```python
from build123d import *

# Parameters (mm, degrees)
CROQUIS1_W              = 208
CROQUIS1_H              = 365
SALIENTE_EXTRUIR1_DEPTH = 2.5
CROQUIS2_W              = 34
CROQUIS2_H              = 30
SALIENTE_EXTRUIR2_DEPTH = 1
CROQUIS3_W              = 208
CROQUIS3_H              = 135
CORTAR_EXTRUIR1_DEPTH   = 4.5
SKETCH1_R               = 2
CUT_EXTRUDE1_DEPTH      = 2.5


with BuildPart() as part:
    # Croquis1 → Saliente-Extruir1 (new body)
    with BuildSketch(Plane(origin=(0, 0, 0), x_dir=(1, 0, 0), z_dir=(0, 1, 0))):
        Rectangle(CROQUIS1_W, CROQUIS1_H)
    extrude(amount=SALIENTE_EXTRUIR1_DEPTH)

    # Croquis2 → Saliente-Extruir2 (add)
    with BuildSketch(Plane(origin=(0, 0, 0), x_dir=(-1, 0, 0), z_dir=(0, -1, 0))):
        with Locations((87, -31.5)):
            Rectangle(CROQUIS2_W, CROQUIS2_H)
        with Locations((-87, -31.5)):
            Rectangle(CROQUIS2_W, CROQUIS2_H)
        with Locations((-87, 22.5)):
            Rectangle(CROQUIS2_W, CROQUIS2_H)
        with Locations((87, 22.5)):
            Rectangle(CROQUIS2_W, CROQUIS2_H)
    extrude(amount=SALIENTE_EXTRUIR2_DEPTH)

    # Croquis3 → Cortar-Extruir1 (cut, through all)
    with BuildSketch(Plane(origin=(0, 2.5, 0), x_dir=(1, 0, 0), z_dir=(0, 1, 0))):
        with Locations((0, 115)):
            Rectangle(CROQUIS3_W, CROQUIS3_H)
    extrude(amount=-CORTAR_EXTRUIR1_DEPTH, mode=Mode.SUBTRACT)

    # Sketch1 → Cut-Extrude1 (cut)
    with BuildSketch(Plane.XZ):
        with Locations((-99, 40.5)):
            Circle(SKETCH1_R)
        with Locations((-75, 40.5)):
            Circle(SKETCH1_R)
        with Locations((-99, 22.5)):
            Circle(SKETCH1_R)
        with Locations((-75, 22.5)):
            Circle(SKETCH1_R)
        with Locations((-99, -13.5)):
            Circle(SKETCH1_R)
        with Locations((-99, -31.5)):
            Circle(SKETCH1_R)
        with Locations((-75, -31.5)):
            Circle(SKETCH1_R)
        with Locations((-75, -13.5)):
            Circle(SKETCH1_R)
        with Locations((75, -13.5)):
            Circle(SKETCH1_R)
        with Locations((75, -31.5)):
            Circle(SKETCH1_R)
        with Locations((99, -31.5)):
            Circle(SKETCH1_R)
        with Locations((99, -13.5)):
            Circle(SKETCH1_R)
        with Locations((99, 22.5)):
            Circle(SKETCH1_R)
        with Locations((75, 22.5)):
            Circle(SKETCH1_R)
        with Locations((75, 40.5)):
            Circle(SKETCH1_R)
        with Locations((99, 40.5)):
            Circle(SKETCH1_R)
        with Locations((-12, 13.5)):
            Circle(SKETCH1_R)
        with Locations((-12, -4.5)):
            Circle(SKETCH1_R)
        with Locations((12, -4.5)):
            Circle(SKETCH1_R)
        with Locations((12, 13.5)):
            Circle(SKETCH1_R)
    extrude(amount=-CUT_EXTRUDE1_DEPTH, mode=Mode.SUBTRACT)


solid = part.part
```
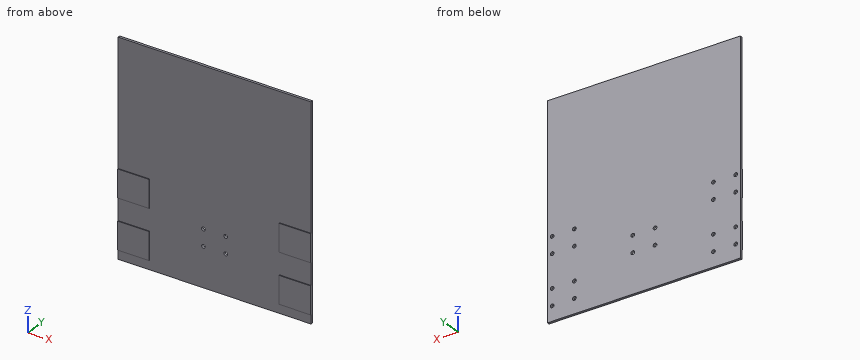
Geometry: final body of the model. Coordinates: model frame, mm. Coordinates: 2 decimals unless noted, no trailing zeros. Order: outer loops, then holes, each group sorted by start corner. A loop starts at its lowest first (then second) coordinate and runs counter-clockwise, first axis right, second up. Notation, with made-up numbers: (-24.75, -3) -> (18.25, -3) arc R3 cw to (18.25, 2) -> close; hole circle Ø8 at (46.5, 46.25). An arc over 180 degrees is marked (long way). Answer in a Markdown table with one row per item.
Item 1: Ray query, L1, parallel to Z at x = 75, y = 1.5; L2, parallel to Z at x = 11, y = 1.6; L3, parallel to Y at x = 52, z = 0.5. Return the intervals inside material, ascending.
Return value:
| item | result |
|---|---|
| L1 | z = -47.5 to -33.5, -29.5 to -15.5, -11.5 to 20.5, 24.5 to 38.5, 42.5 to 182.5 |
| L2 | z = -47.5 to -6.23, -2.77 to 11.77, 15.23 to 182.5 |
| L3 | y = 0 to 2.5 |
Item 2: Contact query for flat-ended pins moving along their axis: P1, Ø1.2, axis at x = -74.5, z = -13, coming from the +Y side; P2, Ø6.5, axis at x = -12, z = -4.5, coming from the -Y side; P3, Ø2.5, axis at x = -12, z = 13.5, coming from the +Y side. Output: stop coordinate, or through.
Return value:
| item | result |
|---|---|
| P1 | stops at y = 0 |
| P2 | stops at y = 0 |
| P3 | passes through |
Item 3: Section A-A on z = -19. Output: boundary loops of the cut face in (x, y).
Return value:
| item | result |
|---|---|
| outline | (-104, -1) -> (-70, -1) -> (-70, 0) -> (70, 0) -> (70, -1) -> (104, -1) -> (104, 2.5) -> (-104, 2.5) -> close |
Item 4: Section C-C on z = 155.5. Output: boundary loops of the cut face in (x, y).
Return value:
| item | result |
|---|---|
| outline | (-104, 0) -> (104, 0) -> (104, 2.5) -> (-104, 2.5) -> close |
Item 5: Section B-B on x = -39.5. Output: boundary loops of the cut face in (y, z), plus the area to 3 significant figures.
Return value:
| item | result |
|---|---|
| outline | (0, -47.5) -> (2.5, -47.5) -> (2.5, 182.5) -> (0, 182.5) -> close |
| area | 575 mm² |
